```python
from build123d import *

# Parameters (mm, degrees)
ESQUISSE1_R             = 2.5
BOSS_EXTRU_1_DEPTH      = 5
ENL_V_MAT_EXTRU_1_DEPTH = 41.47085371
CONG_1_R                = 10


with BuildPart() as part:
    # Esquisse1 → Boss.-Extru.1 (new body)
    with BuildSketch(Plane.XY):
        with BuildLine():
            Line((-7.5, -19.7), (7.5, -19.7))
            ThreePointArc((7.5, -19.7), (8.759622792, -23.860251472), (12.115384615, -26.623076923))
            ThreePointArc((12.115384615, -26.623076923), (13.054700196, -26.532050294), (13.5, -25.7))
            Line((13.5, -25.7), (13.5, -20.7))
            ThreePointArc((13.5, -20.7), (13.792893219, -19.992893219), (14.5, -19.7))
            Line((14.5, -19.7), (15.5, -19.7))
            ThreePointArc((15.5, -19.7), (16.207106781, -19.992893219), (16.5, -20.7))
            Line((16.5, -20.7), (16.5, -25.7))
            ThreePointArc((16.5, -25.7), (16.945299804, -26.532050294), (17.884615385, -26.623076923))
            ThreePointArc((17.884615385, -26.623076923), (21.240377208, -23.860251472), (22.5, -19.7))
            Line((22.5, -19.7), (30, -19.7))
            Line((30, -19.7), (30, 19.7))
            Line((30, 19.7), (22.5, 19.7))
            ThreePointArc((22.5, 19.7), (21.240377208, 23.860251472), (17.884615385, 26.623076923))
            ThreePointArc((17.884615385, 26.623076923), (16.945299804, 26.532050294), (16.5, 25.7))
            Line((16.5, 25.7), (16.5, 20.7))
            ThreePointArc((16.5, 20.7), (16.207106781, 19.992893219), (15.5, 19.7))
            Line((15.5, 19.7), (14.5, 19.7))
            ThreePointArc((14.5, 19.7), (13.792893219, 19.992893219), (13.5, 20.7))
            Line((13.5, 20.7), (13.5, 25.7))
            ThreePointArc((13.5, 25.7), (13.054700196, 26.532050294), (12.115384615, 26.623076923))
            ThreePointArc((12.115384615, 26.623076923), (8.759622792, 23.860251472), (7.5, 19.7))
            Line((7.5, 19.7), (-7.5, 19.7))
            ThreePointArc((-7.5, 19.7), (-8.759622792, 23.860251472), (-12.115384615, 26.623076923))
            ThreePointArc((-12.115384615, 26.623076923), (-13.054700196, 26.532050294), (-13.5, 25.7))
            Line((-13.5, 25.7), (-13.5, 20.7))
            ThreePointArc((-13.5, 20.7), (-13.792893219, 19.992893219), (-14.5, 19.7))
            Line((-14.5, 19.7), (-15.5, 19.7))
            ThreePointArc((-15.5, 19.7), (-16.207106781, 19.992893219), (-16.5, 20.7))
            Line((-16.5, 20.7), (-16.5, 25.7))
            ThreePointArc((-16.5, 25.7), (-16.945299804, 26.532050294), (-17.884615385, 26.623076923))
            ThreePointArc((-17.884615385, 26.623076923), (-21.240377208, 23.860251472), (-22.5, 19.7))
            Line((-22.5, 19.7), (-30, 19.7))
            Line((-30, 19.7), (-30, -19.7))
            Line((-30, -19.7), (-22.5, -19.7))
            ThreePointArc((-22.5, -19.7), (-21.240377208, -23.860251472), (-17.884615385, -26.623076923))
            ThreePointArc((-17.884615385, -26.623076923), (-16.945299804, -26.532050294), (-16.5, -25.7))
            Line((-16.5, -25.7), (-16.5, -20.7))
            ThreePointArc((-16.5, -20.7), (-16.207106781, -19.992893219), (-15.5, -19.7))
            Line((-15.5, -19.7), (-14.5, -19.7))
            ThreePointArc((-14.5, -19.7), (-13.792893219, -19.992893219), (-13.5, -20.7))
            Line((-13.5, -20.7), (-13.5, -25.7))
            ThreePointArc((-13.5, -25.7), (-13.054700196, -26.532050294), (-12.115384615, -26.623076923))
            ThreePointArc((-12.115384615, -26.623076923), (-8.759622792, -23.860251472), (-7.5, -19.7))
        make_face()
        Circle(ESQUISSE1_R, mode=Mode.SUBTRACT)
    extrude(amount=BOSS_EXTRU_1_DEPTH)

    # Esquisse2 → Enlèv. mat.-Extru.1 (cut, through all)
    with BuildSketch(Plane.XY.offset(5)):
        with BuildLine():
            Line((-30, 12.741190179), (-30, -12.741190179))
            ThreePointArc((-30, -12.741190179), (-22.915937899, 0), (-30, 12.741190179))
        make_face()
        with BuildLine():
            Line((30, 12.741190179), (30, -12.741190179))
            ThreePointArc((30, -12.741190179), (22.915937899, 0), (30, 12.741190179))
        make_face()
    extrude(amount=-ENL_V_MAT_EXTRU_1_DEPTH, mode=Mode.SUBTRACT)

    # Congé1
    cong_1_edges = [part.edges().sort_by_distance(p)[0] for p in [
        (-30, 12.741190179, 2.5),
        (-30, -12.741190179, 2.5),
        (30, -12.741190179, 2.5),
        (30, 12.741190179, 2.5),
    ]]
    fillet(cong_1_edges, radius=CONG_1_R)


solid = part.part
```
CAD build for the part. Positions are in the model's coordinates, mm. A direction names the side the tool comes from. Coordinates: 2 decimals unless noted, no trailing zeros. Order: outer loops, then holes, each group sorted by start corner. A loop starts at its lowest first (then second) coordinate and runs counter-clockwise, first axis right, second up. Notation, with made-up numbers: (-17.5, 22.25) -> (37.5, 22.25) arc R14 ccw to (37.5, 43.25) -> close; hole circle Ø4 at (13.5, -7). An arc over 180 degrees is marked (long way). Use one line per item in the form item = value. Start each with the question number.
1) Drill centre lines: L1, parallel to Y at x = 0, z = 2.8; L2, parallel to X at y = 24.5, z = 3.4; L3, parallel to X at y = -20.5, z = 2.75. Where is each one in solid material? Low to high. Write a range as [from, to].
2) Pull direction X, two halves, no side cores. Call faces 1 (the flat face through (16.5, -23, 2)), 2 (the cylindrical face through (-22.917, -0.162, 2.535)), 3 (the flat face through (26, -19.7, 2)): +X half, -X half, draft (parallel to the pull), parting line (faces both ways), or undercut.
3) Drop flat-ended pins along their axis: pin 1 (1.5 mm diameter, centred on y = 0, z = 4.5, fed in from -X); pin 2 (2.5 mm diameter, centred on x = -26, z = 2, fed in from +Y); pin 3 (1.5 mm diameter, centred on y = 23, z = 2.5, fed in from -X); pin 4 (12 mm diameter, centred on x = 15, y = 6, fed in from -Z). Give the stop position or say it passes through.
4) Band-saw the part on C-C on y = 7. Give the cut face in (x, z).
5) Band-saw the part on B-B on y = 0. Give the cut face in (x, z).
6) Tool access for faces 4 (the flat face through (-26, 19.7, 2)), 5 (the cylindrical face through (-29.285, -13.722, 2.465)), 6 (the flat face through (-16.5, -23, 2)), 7 (the cylindrical face through (-8.726, 23.809, 2.465)): list every direction of +Z, -Z, +X, -X, +Y, -Y with a clear straight run to the whole face (end or side of a thin tool).
7) Band-saw the part on A-A on x = 0. Give the cut face in (y, z), then the cut area to 3 significant figures.
Entries:
q1.L1 = [-19.7, -2.5], [2.5, 19.7]
q1.L2 = [-20.76, -16.5], [-13.5, -9.24], [9.24, 13.5], [16.5, 20.76]
q1.L3 = [-22.46, -16.48], [-13.52, -7.54], [7.54, 13.52], [16.48, 22.46]
q2.face_1 = undercut
q2.face_2 = -X half
q2.face_3 = draft
q3.pin_1 = -22.93
q3.pin_2 = 19.7
q3.pin_3 = -22.05
q3.pin_4 = 0
q4.outline = (-24.65, 0) -> (24.65, 0) -> (24.65, 5) -> (-24.65, 5) -> close
q5.outline = (-22.92, 0) -> (-2.5, 0) -> (-2.5, 5) -> (-22.92, 5) -> close; (2.5, 0) -> (22.92, 0) -> (22.92, 5) -> (2.5, 5) -> close
q6.face_4 = +Z, -Z, -X, +Y
q6.face_5 = +Z, -Z, -X
q6.face_6 = +Z, -Z, -Y
q6.face_7 = +Z, -Z, +Y
q7.outline = (-19.7, 0) -> (-2.5, 0) -> (-2.5, 5) -> (-19.7, 5) -> close; (2.5, 0) -> (19.7, 0) -> (19.7, 5) -> (2.5, 5) -> close
q7.area = 172 mm2
